from build123d import *

# Parameters (mm, degrees)
BASE_FLANGE1_DEPTH  = 25.4
SKETCH7_W           = 41.275
SKETCH7_H           = 19.05
BOSS_EXTRUDE1_DEPTH = 3.175
SKETCH6_R           = 2.45745
SKETCH6_R_2         = 4.3688
CUT_EXTRUDE1_DEPTH  = 58.474902009
CUT_EXTRUDE2_DEPTH  = 58.474902009
FILLET1_R           = 3.175


# Sheet-metal steps are written as plain solids
with BuildPart() as part:
    # Sketch1 → Base-Flange1 (new, symmetric)
    with BuildSketch(Plane.XY):
        with BuildLine():
            Line((0, 0), (22.225, 0))
            ThreePointArc((22.225, 0), (24.47006403, -0.92993597), (25.4, -3.175))
            Line((25.4, -3.175), (25.4, -16.256))
            ThreePointArc((25.4, -16.256), (24.47006403, -18.50106403), (22.225, -19.431))
            Line((22.225, -19.431), (-22.225, -19.431))
            Line((-22.225, -19.431), (-22.225, -22.606))
            Line((-22.225, -22.606), (22.225, -22.606))
            ThreePointArc((22.225, -22.606), (26.715128061, -20.746128061), (28.575, -16.256))
            Line((28.575, -16.256), (28.575, -3.175))
            ThreePointArc((28.575, -3.175), (26.715128061, 1.315128061), (22.225, 3.175))
            Line((22.225, 3.175), (0, 3.175))
            Line((0, 3.175), (0, 0))
        make_face()
    extrude(amount=BASE_FLANGE1_DEPTH, both=True)

    # Sketch7 → Boss-Extrude1 (add)
    with BuildSketch(Plane.XZ.offset(22.606)):
        with Locations((-1.5875, 34.925)):
            Rectangle(SKETCH7_W, SKETCH7_H)
        with Locations((-1.5875, -34.925)):
            Rectangle(SKETCH7_W, SKETCH7_H)
    extrude(amount=-BOSS_EXTRUDE1_DEPTH)

    # Sketch6 → Cut-Extrude1 (cut, through all)
    with BuildSketch(Plane(origin=(0, -19.431, 0), x_dir=(1, 0, 0), z_dir=(0, 1, 0))):
        with Locations(Location((-13.7668, 12.7, 0), (0, 0, 180))):
            Circle(SKETCH6_R)
        with Locations(Location((-13.7668, -12.7, 0), (0, 0, 180))):
            Circle(SKETCH6_R)
        with Locations(Location((10.287, -34.925, 0), (0, 0, 180))):
            Circle(SKETCH6_R_2)
        with Locations(Location((10.287, 34.925, 0), (0, 0, 180))):
            Circle(SKETCH6_R_2)
    extrude(amount=-CUT_EXTRUDE1_DEPTH, mode=Mode.SUBTRACT)

    # Sketch8 → Cut-Extrude2 (cut, through all)
    with BuildSketch(Plane(origin=(0, -19.431, 0), x_dir=(1, 0, 0), z_dir=(0, 1, 0))):
        Polygon((0, -44.45), (-22.225, -25.4), (-22.225, -44.45), align=None)
        Polygon((-22.225, 44.45), (-22.225, 25.4), (0, 44.45), align=None)
    extrude(amount=-CUT_EXTRUDE2_DEPTH, mode=Mode.SUBTRACT)

    # Fillet1
    fillet1_edges = [part.edges().sort_by_distance(p)[0] for p in [
        (0, 1.5875, -25.4),
        (0, 1.5875, 25.4),
        (19.05, -21.0185, -25.4),
        (19.05, -21.0185, -44.45),
        (19.05, -21.0185, 25.4),
        (19.05, -21.0185, 44.45),
        (0, -21.0185, 44.45),
        (-22.225, -21.0185, 25.4),
        (0, -21.0185, -44.45),
        (-22.225, -21.0185, -25.4),
    ]]
    fillet(fillet1_edges, radius=FILLET1_R)


solid = part.part
Geometry: final body of the model. Coordinates: model frame, mm. A direction names the side the tool comes from. Give positions to 0.01 mm unless a question says otherwise; leave off trailing zeros. Write each loop counter-clockwise with the first axis right and the second up, starting at its lowest first coordinate (ties: lowest second). Pieces come first, ordered by that corner, then holes. Notation, with made-up numbers: M 56.5,15.25 L 87.5,15.25 A19 cw 87.5,26.25 Z; hole C 6.5,41.5 d3. An arc over 180 degrees is marked long. Answer in a Markdown table with one row per item. Add a question column.
(1) Ray query, line 1 (Y direction, x = 17, z = 15) (3 decimals); line 2 (X direction, y = -9.25, z = -24.5) (3 decimals); line 3 (Y direction, x = -4.5, z = 28.5). Return the intervals inside material, ascending.
(2) Section A-A on z = 12.7. Return loops of the section in (x, y) (3 decimals).
(3) First-contact query: pin 1 (1.5 mm diameter, centred on y = -19, z = -24.5, fed in from +X); pin 2 (12 mm diameter, centred on x = -17, z = 19, fed in from +Y); pin 3 (11.5 mm diameter, centred on x = 10.287, z = -34.925, fed in from -Y); pin 4 (3.5 mm diameter, centred on y = -20.5, z = -37.5, fed in from +X). Flat tips, straight axial feed; report the tip coordinate or a pass-through.
(4) Section C-C on z = -37.5. Return loops of the section in (x, y).
(5) Section D-D on y = -8.25. Return loops of the section in (x, z) (3 decimals).
(6) Reachability of faces 1 (the flat face through (19.05, -21, -35)), 2 (the cylindrical face through (24.49, -18.48, 0.36)), 3 (the flat face through (0, 2, 0)), 4 (the flat face through (19.05, -21, 35)) from +Z, -Z, +X, -X, +Y, -Y: full face, straight path, thin tool, end or side. Return the list, or none.
(7) Mould query, pull axis Z, two halves, no side actions, for faces 5 (the flat face through (0, -22.606, 1)), 6 (the cylindrical face through (-14.9, -21, -14.88)), 7 (the cylindrical face through (-21.94, -21.04, 25.25)). Classes: +Z half, -Z half, draft (parallel to the pull), parting line (faces both ways), or undercut.
(8) Section B-B on x = 7. Return loops of the section in (y, z) (3 decimals), and give its area (3 significant figures).
Result set:
| question | item | result |
|---|---|---|
| 1 | line 1 | y = -22.606 to -19.431, 0 to 3.175 |
| 1 | line 2 | x = 25.4 to 28.575 |
| 1 | line 3 | y = -22.61 to -19.43 |
| 2 | outline | M -22.225,-22.606 L -16.224,-22.606 L -16.224,-19.431 L -22.225,-19.431 Z; M -11.309,-22.606 L 22.225,-22.606 A6.35 ccw 28.575,-16.256 L 28.575,-3.175 A6.35 ccw 22.225,3.175 L 0,3.175 L 0,0 L 22.225,0 A3.175 cw 25.4,-3.175 L 25.4,-16.256 A3.175 cw 22.225,-19.431 L -11.309,-19.431 Z |
| 3 | pin 1 | stops at x = 28.25 |
| 3 | pin 2 | stops at y = -19.43 |
| 3 | pin 3 | stops at y = -22.61 |
| 3 | pin 4 | stops at x = 19.05 |
| 4 | outline | M -8.11,-22.61 L 6.76,-22.61 L 6.76,-19.43 L -8.11,-19.43 Z; M 13.82,-22.61 L 19.05,-22.61 L 19.05,-19.43 L 13.82,-19.43 Z |
| 5 | outline | M 25.4,-25.4 L 28.575,-25.4 L 28.575,25.4 L 25.4,25.4 Z |
| 6 | face 1 | -Z, +X, +Y, -Y |
| 6 | face 2 | +Z, -Z, -X |
| 6 | face 3 | +Z, -Z, -X, +Y |
| 6 | face 4 | +Z, +X, +Y, -Y |
| 7 | face 5 | draft |
| 7 | face 6 | undercut |
| 7 | face 7 | +Z half |
| 8 | outline | M -22.606,-44.45 L -19.431,-44.45 L -19.431,-37.803 L -22.606,-37.803 Z; M -22.606,-32.047 L -19.431,-32.047 L -19.431,32.047 L -22.606,32.047 Z; M -22.606,37.803 L -19.431,37.803 L -19.431,44.45 L -22.606,44.45 Z; M 0,-25.4 L 3.175,-25.4 L 3.175,25.4 L 0,25.4 Z |
| 8 | area | 407 mm^2 |
